Verification items for this drawing (mm, ordinates from the low corner). A direction names the side the tool comes from. Give positions to 0.01 mm unless a question says otherwise; leave off trailing zeros. Write each loop counter-clockwise with the first axis right and the second up, starting at its lowest first coordinate (ties: lowest second). Pieces come first, ordered by that corner, then holes. Notation, with made-up numbers: (59, 71.25) -> (89, 71.25) arc R21 cw to (89, 94.25) -> close; hole circle Ø5 at (27.5, -7). An arc over 180 degrees is marked (long way). One line per item, written item: value.
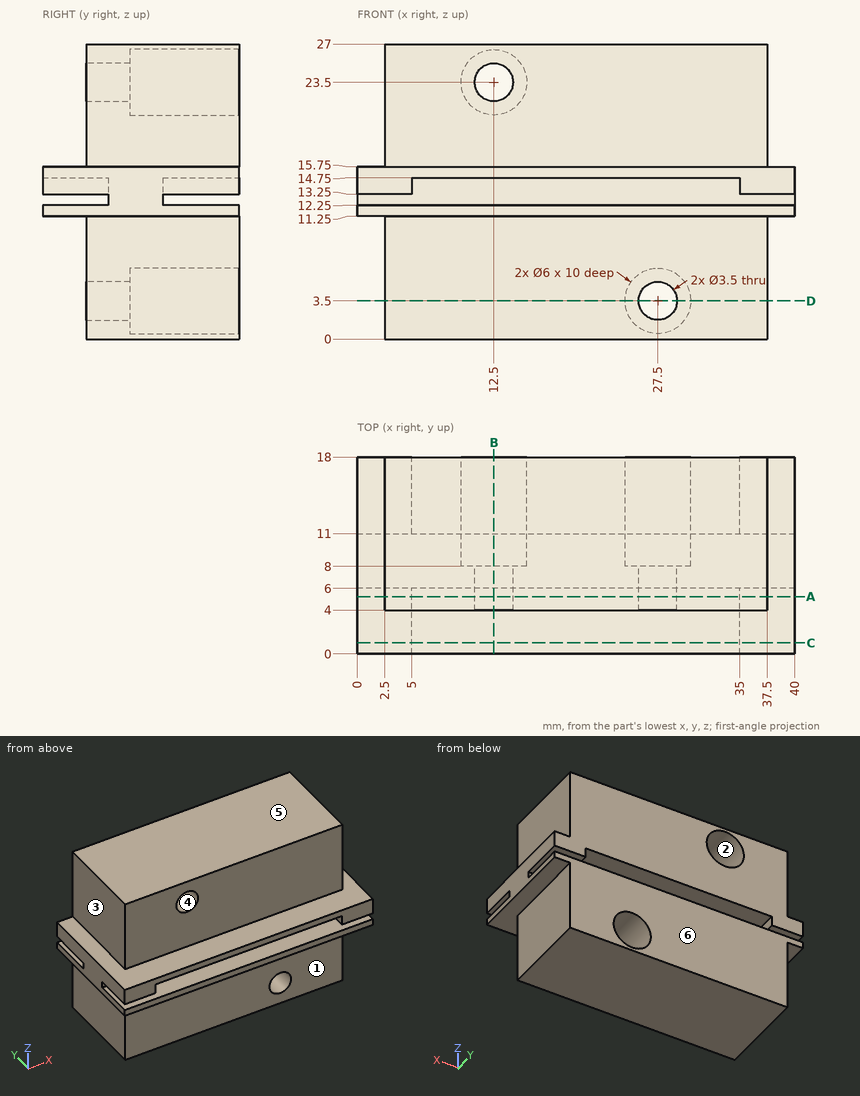
1) Sectioned sample at C-C on y = 1. Record the cut outline in (x, z).
Verdict:
outline: (0, 11.25) -> (40, 11.25) -> (40, 12.25) -> (0, 12.25) -> close; (0, 13.25) -> (5, 13.25) -> (5, 14.75) -> (35, 14.75) -> (35, 13.25) -> (40, 13.25) -> (40, 15.75) -> (0, 15.75) -> close
2) Sectioned sample at A-A on y = 5.25. Record the cut outline in (x, z).
Verdict:
outline: (0, 11.25) -> (2.5, 11.25) -> (2.5, 0) -> (37.5, 0) -> (37.5, 11.25) -> (40, 11.25) -> (40, 12.25) -> (0, 12.25) -> close; (0, 13.25) -> (5, 13.25) -> (5, 14.75) -> (35, 14.75) -> (35, 13.25) -> (40, 13.25) -> (40, 15.75) -> (37.5, 15.75) -> (37.5, 27) -> (2.5, 27) -> (2.5, 15.75) -> (0, 15.75) -> close; hole circle Ø3.5 at (12.5, 23.5); hole circle Ø3.5 at (27.5, 3.5)
3) Tool access check on the marked faces 1, 2 and 3. Record the directions out of +Z, -Z, +X, -X, +Y, -Y that give a thin tool (end or side, any length) a straight path to the whole face; none if there is none.
Verdict:
face 1: -Z, +X, -X, -Y
face 2: +Y
face 3: +Z, -X, +Y, -Y
4) Mould release check, pull along Z, two halves, no side actions. Record for the marked faces 4, 5 and 6: released by +Z, released by -Z, zero draft, split by the parting line, or undercut.
Verdict:
face 4: undercut
face 5: released by +Z
face 6: zero draft
5) Scan lines: probe 1 along Z at (x, y) = (17, 15.5); probe 2 along X at (y, z) = (11.5, 23.5); probe 3 along X at (y, z) = (7.15, 3.5). Record each from-to range of solid material in increasing order.
Verdict:
probe 1: 0 to 12.25, 14.75 to 27
probe 2: 2.5 to 9.5, 15.5 to 37.5
probe 3: 2.5 to 25.75, 29.25 to 37.5
6) Depth check by flat-ended pin: pin 1 Ø3.5 at (x, z) = (14.5, 20.5) entering from -Y; pin 2 Ø6 at (y, z) = (6, 6.5) entering from -X; pin 3 Ø1.5 at (x, y) = (38.5, 3) entering from -Z. Enter the tip coordinate at first touch or a pass-through.
Verdict:
pin 1: y = 4
pin 2: x = 2.5
pin 3: z = 11.25
7) Sectioned sample at D-D on z = 3.5. Record the cut outline in (x, y), plus the area to 3 significant figures.
Verdict:
outline: (2.5, 4) -> (25.75, 4) -> (25.75, 8) -> (24.5, 8) -> (24.5, 18) -> (2.5, 18) -> close; (29.25, 4) -> (37.5, 4) -> (37.5, 18) -> (30.5, 18) -> (30.5, 8) -> (29.25, 8) -> close
area: 416 mm^2
8) Sectioned sample at B-B on x = 12.5. Record the cut outline in (y, z).
Verdict:
outline: (0, 11.25) -> (4, 11.25) -> (4, 0) -> (18, 0) -> (18, 12.25) -> (11, 12.25) -> (11, 14.75) -> (18, 14.75) -> (18, 20.5) -> (8, 20.5) -> (8, 21.75) -> (4, 21.75) -> (4, 15.75) -> (0, 15.75) -> (0, 14.75) -> (6, 14.75) -> (6, 12.25) -> (0, 12.25) -> close; (4, 25.25) -> (8, 25.25) -> (8, 26.5) -> (18, 26.5) -> (18, 27) -> (4, 27) -> close
